```python
from build123d import *

# Parameters (mm, degrees)
BOSS_EXTRUDE1_DEPTH = 241.3
SKETCH2_R           = 63.5
CUT_EXTRUDE1_DEPTH  = 482.6
SKETCH4_R           = 12.7
CUT_EXTRUDE3_DEPTH  = 120.65
RIB1_START          = -120.65
RIB1_DEPTH          = 120.65
RIB2_REACH          = 371.169
RIB3_REACH          = 371.169
SKETCH7_WALLS_W     = 749.266761297
SKETCH7_WALLS_H     = 5


# Read off the part's stored shape, not the designer's step: Rib1
with BuildPart() as part:
    # Sketch1 → Boss-Extrude1 (new, symmetric)
    with BuildSketch(Plane(origin=(0, 0, 0), x_dir=(0, 0, -1), z_dir=(1, 0, 0))):
        with BuildLine():
            Line((0, 175.36), (58.62, 175.36))
            Line((58.62, 175.36), (139.636486112, 256.376486112))
            Line((139.636486112, 256.376486112), (255.494783215, 138.754783215))
            Line((255.494783215, 138.754783215), (165.1, 48.36))
            Line((165.1, 48.36), (165.1, 0))
            Line((165.1, 0), (63.5, 0))
            ThreePointArc((63.5, 0), (44.901280605, 44.901280605), (0, 63.5))
            Line((0, 63.5), (0, 175.36))
        make_face()
    extrude(amount=BOSS_EXTRUDE1_DEPTH, both=True)

    # Sketch2 → Cut-Extrude1 (cut)
    with BuildSketch(Plane(origin=(0, 196.062295457, -199.046435538), x_dir=(-1, 0, 0), z_dir=(0, 0.7017461968633759, -0.7124270314830763))):
        with Locations(Location((-146.05, 2.11016587, 0), (0, 0, 90))):
            Circle(SKETCH2_R)
        with Locations(Location((0, 2.11016587, 0), (0, 0, 90))):
            Circle(SKETCH2_R)
        with Locations(Location((146.05, 2.11016587, 0), (0, 0, 90))):
            Circle(SKETCH2_R)
    extrude(amount=-CUT_EXTRUDE1_DEPTH, mode=Mode.SUBTRACT)

    # Sketch4 → Cut-Extrude3 (cut)
    # profile 1 of 3: a face of its own
    with BuildSketch(Plane(origin=(0, 196.062295457, -199.046435538), x_dir=(-1, 0, 0), z_dir=(0, 0.7017461968632962, -0.7124270314831548))):
        with BuildLine():
            Line((-228.6, -62.166812966), (-228.6, -67.73983413))
            Line((-228.6, -67.73983413), (-176.503530173, -67.73983413))
            ThreePointArc((-176.503530173, -67.73983413), (-222.25, 2.11016587), (-176.503530173, 71.96016587))
            Line((-176.503530173, 71.96016587), (-228.6, 71.96016587))
            Line((-228.6, 71.96016587), (-228.6, 66.387144707))
            ThreePointArc((-228.6, 66.387144707), (-214.584025044, 69.870701255), (-206.372106927, 57.99016587))
            ThreePointArc((-206.372106927, 57.99016587), (-214.584025044, 46.109630486), (-228.6, 49.593187034))
            Line((-228.6, 49.593187034), (-228.6, -45.372855293))
            ThreePointArc((-228.6, -45.372855293), (-214.584025044, -41.889298745), (-206.372106927, -53.76983413))
            ThreePointArc((-206.372106927, -53.76983413), (-214.584025044, -65.650369514), (-228.6, -62.166812966))
        make_face()
    # profile 2 of 3: a face of its own
    with BuildSketch(Plane(origin=(0, 196.062295457, -199.046435538), x_dir=(-1, 0, 0), z_dir=(0, 0.7017461968632962, -0.7124270314831548))):
        with BuildLine():
            Line((-30.453530173, 71.96016587), (-115.596469827, 71.96016587))
            ThreePointArc((-115.596469827, 71.96016587), (-88.997809808, 52.622417793), (-73.025, 23.876869227))
            ThreePointArc((-73.025, 23.876869227), (-57.052190192, 52.622417793), (-30.453530173, 71.96016587))
        make_face()
        with Locations(Location((-73.027893073, 57.99016587, 0), (0, 0, 90))):
            Circle(SKETCH4_R, mode=Mode.SUBTRACT)
    # profile 3 of 3: a face of its own
    with BuildSketch(Plane(origin=(0, 196.062295457, -199.046435538), x_dir=(-1, 0, 0), z_dir=(0, 0.7017461968632962, -0.7124270314831548))):
        with BuildLine():
            ThreePointArc((-73.025, -19.656537486), (-88.997809808, -48.402086052), (-115.596469827, -67.73983413))
            Line((-115.596469827, -67.73983413), (-30.453530173, -67.73983413))
            ThreePointArc((-30.453530173, -67.73983413), (-57.052190192, -48.402086052), (-73.025, -19.656537486))
        make_face()
        with Locations(Location((-73.027893073, -53.76983413, 0), (0, 0, 90))):
            Circle(SKETCH4_R, mode=Mode.SUBTRACT)
    extrude(amount=-CUT_EXTRUDE3_DEPTH, mode=Mode.SUBTRACT)

    # Rib1 outline → Rib1 (add)
    with BuildSketch(Plane(origin=(0, 196.062295457, -199.046435538), x_dir=(-1, 0, 0), z_dir=(0, 0.7017461968632962, -0.7124270314831548)).offset(RIB1_START)):
        with BuildLine():
            ThreePointArc((-85.252237114, -43.825354461), (-86.81154021, -45.819416661), (-88.436216043, -47.760586061))
            Line((-88.436216043, -47.760586061), (-85.061213526, -49.709144673))
            ThreePointArc((-85.061213526, -49.709144673), (-84.026415701, -47.41983413), (-82.561213527, -45.379017654))
            Line((-82.561213527, -45.379017654), (-85.252237114, -43.825354461))
        make_face()
        with BuildLine():
            ThreePointArc((-70.527893073, -66.221340063), (-73.027893073, -66.46983413), (-75.527893073, -66.221340063))
            Line((-75.527893073, -66.221340063), (-75.527893073, -67.73983413))
            Line((-75.527893073, -67.73983413), (-70.527893073, -67.73983413))
            Line((-70.527893073, -67.73983413), (-70.527893073, -66.221340063))
        make_face()
    extrude(amount=RIB1_DEPTH)

    # Sketch6 walls → Rib2 (add, up to next)
    with BuildSketch(Plane(origin=(0, 196.062295457, -199.046435538), x_dir=(-1, 0, 0), z_dir=(0, 0.7017461968632962, -0.7124270314831548)), mode=Mode.PRIVATE) as rib2_sk1:
        Polygon((-365.486871932, -280.7035923), (235.169541879, 178.910932933), (232.131085785, 182.881799912), (-368.525328026, -276.732725322), align=None)
    rib2_tool1 = extrude(rib2_sk1.sketch, amount=-RIB2_REACH, mode=Mode.PRIVATE) - part.part
    add(rib2_tool1.solids().sort_by_distance((66.677893073, 161.216850874, -233.369470927))[0])

    # Sketch7 walls → Rib3 (add, up to next)
    with BuildSketch(Plane(origin=(0, 196.062295457, -199.046435538), x_dir=(-1, 0, 0), z_dir=(0, 0.7017461968632962, -0.7124270314831548)), mode=Mode.PRIVATE) as rib3_sk1:
        with Locations((-201.90751874, -53.76983413)):
            Rectangle(SKETCH7_WALLS_W, SKETCH7_WALLS_H)
    rib3_tool1 = extrude(rib3_sk1.sketch, amount=-RIB3_REACH, mode=Mode.PRIVATE) - part.part
    add(rib3_tool1.solids().sort_by_distance((201.907518739, 157.755212144, -236.779212144))[0])


solid = part.part
```
Here's how the part is built. I have some questions about the finished solid (model axes, mm). A direction names the side the tool comes from. Give positions to 0.01 mm unless a question says otherwise; leave off trailing zeros. Loops run counter-clockwise (first coordinate to the right, second up) from the corner with the lowest first, then second, coordinate; pieces in that order, holes last. Notation, with made-up numbers: (-5, 75.5) -> (48, 75.5) arc R8 ccw to (48, 83.5) -> close; hole circle Ø4 at (9.25, 25). An arc over 180 degrees is marked (long way). Use one line per item in the form item = value. Start each with the question number.
1) Imagine slicing it at C-C (x = -173). Please give me the cut outline in (y, z).
2) For P1, Ø8, axis at x = -123.5, y = 154.5, coming from the -Z side; P2, Ø5, axis at x = 54, z = -169, coming from the +Y side; P3, Ø17.5, axis at x = -91, z = -34, coming from the +Y side; P4, Ø1, axis at x = 120.5, y = 157.5, coming from the +Z side, each with a flat end and sliding along its axis, tell me the tip position at first contact or that it passes through.
3) Which directions (+Z, -Z, +X, -X, +Y, -Y) give clear straight access to the entire face, cutting with the end or side of a thin tool? Please do faces 5 (the face through (60.311, 120.705, -189.784)), 6 (the face through (73.445, 44.405, -45.392)).
4) Imagine slicing it at A-A (x = -20). Please give me the cut outline in (y, z).
5) Thinking about a two-plate mould opening in X: for faces 1 (the face through (3.38, 215.3, -98.56)), 2 (the face through (-241.3, 130, -130)), 3 (the face through (221.043, 165.449, -145.711)), 4 (the face through (72.429, 205.588, -106.173)), which applies, +X half, -X half, draft (parallel to the pull), parting line (faces both ways), or undercut?
6) Please list where these lines run through material, in increasing order: line 1 along X through (y, z) = (121.5, -125); line 2 along Z through (x, y) = (179, 142.5); line 3 along X through (y, z) = (207, -147).
7) Imagine slicing it at B-B (y = 208). Count the separate pieces of the cut face and the enclosed holes in it, then the cut area to 3 significant figures.
Check values:
q1.outline = (0, -165.1) -> (48.36, -165.1) -> (138.75, -255.49) -> (156.6, -237.91) -> (0, -78.93) -> close; (83.67, 0) -> (238.53, -157.22) -> (256.38, -139.64) -> (175.36, -58.62) -> (175.36, 0) -> close
q2.P1 = -243.93
q2.P2 = 229.1
q2.P3 = 175.36
q2.P4 = 0
q3.face_5 = none
q3.face_6 = +Z, +X, -X, -Y
q4.outline = (0, -165.1) -> (48.36, -165.1) -> (138.75, -255.49) -> (154.63, -239.86) -> (0, -82.88) -> close; (87.56, 0) -> (240.5, -155.27) -> (256.38, -139.64) -> (175.36, -58.62) -> (175.36, 0) -> close
q5.face_1 = draft
q5.face_2 = -X half
q5.face_3 = undercut
q5.face_4 = undercut
q6.line_1 = -241.3 to -209.47, -82.63 to -63.42, 63.42 to 82.63, 209.47 to 222.18, 228.6 to 241.3
q6.line_2 = -251.81 to -241.2, -239.57 to -219.01, -64.31 to 0
q6.line_3 = -241.3 to -193.49, -98.61 to -47.44, 47.44 to 63.44, 82.61 to 98.61, 193.49 to 209.49, 228.6 to 241.3
q7.separate_pieces = 2
q7.enclosed_holes = 1
q7.area = 24,700 mm^2
